Check sheet for the modelled part. Datum: model origin and axes. Units: mm. Face numbers are marked on the shaded views. A direction names the side the tool comes from. Round coordinates to 2 decimals unless told otherwise and drop trailing zeros. Write each loop counter-clockwise with the first axis right and the second up, starting at its lowest first coordinate (ties: lowest second). Pieces come first, ordered by that corner, then holes. Notation, with made-up numbers: M 21.25,87 L 49.25,87 A30 ccw 49.25,114 Z; hole C -40,13.5 d7. An arc over 180 degrees is marked long. One line per item, written item: value.
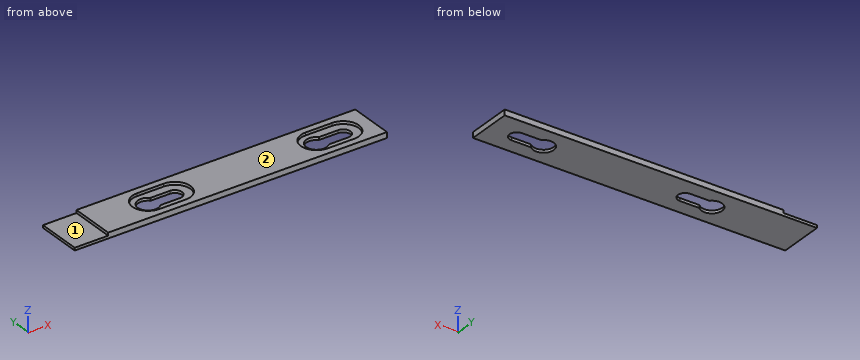
from build123d import *

# Parameters (mm, degrees)
SKETCH_W        = 140
SKETCH_H        = 20
PAD_DEPTH       = 2.5
SKETCH001_W     = 15
SKETCH001_H     = 20
POCKET_DEPTH    = 1.3
POCKET001_DEPTH = 1.25
SKETCH003_R     = 4.6
POCKET002_DEPTH = 1.251


with BuildPart() as part:
    # Sketch → Pad (new body)
    with BuildSketch(Plane.XY):
        with Locations((72, 12)):
            Rectangle(SKETCH_W, SKETCH_H)
    extrude(amount=PAD_DEPTH)

    # Sketch001 → Pocket (cut)
    with BuildSketch(Plane.XY.offset(2.5)):
        with Locations((9.5, 12)):
            Rectangle(SKETCH001_W, SKETCH001_H)
    extrude(amount=-POCKET_DEPTH, mode=Mode.SUBTRACT)

    # Sketch002 → Pocket001 (cut)
    with BuildSketch(Plane.XY.offset(2.5)):
        with BuildLine():
            ThreePointArc((42, 19), (35, 12), (42, 5))
            Line((42, 5), (54, 5))
            ThreePointArc((54, 5), (61, 12), (54, 19))
            Line((42, 19), (54, 19))
        make_face()
        with BuildLine():
            ThreePointArc((117.5, 19), (110.5, 12), (117.5, 5))
            Line((117.5, 5), (129.5, 5))
            ThreePointArc((129.5, 5), (136.5, 12), (129.5, 19))
            Line((117.5, 19), (129.5, 19))
        make_face()
    extrude(amount=-POCKET001_DEPTH, mode=Mode.SUBTRACT)

    # Sketch003 → Pocket002 (cut, through all)
    with BuildSketch(Plane.XY.offset(1.25)):
        with Locations((42, 12)):
            Circle(SKETCH003_R)
        with Locations((117.5, 12)):
            Circle(SKETCH003_R)
        with BuildLine():
            ThreePointArc((54, 8.8), (57.2, 12), (54, 15.2))
            Line((54, 15.2), (44, 15.2))
            ThreePointArc((44, 15.2), (40.8, 12), (44, 8.8))
            Line((54, 8.8), (44, 8.8))
        make_face()
        with BuildLine():
            ThreePointArc((129.5, 8.8), (132.7, 12), (129.5, 15.2))
            Line((129.5, 15.2), (119.5, 15.2))
            ThreePointArc((119.5, 15.2), (116.3, 12), (119.5, 8.8))
            Line((129.5, 8.8), (119.5, 8.8))
        make_face()
    extrude(amount=-POCKET002_DEPTH, mode=Mode.SUBTRACT)


solid = part.part
Q1. Scan lines: line 1 (X direction, y = 12, z = 0.85); line 2 (X direction, y = 13, z = 0.9); line 3 (Y direction, x = 117.5, z = 0.9). Record each from-to range of solid material in increasing order. Write a range as [from, to].
Completed:
line 1: [2, 37.4], [57.2, 112.9], [132.7, 142]
line 2: [2, 37.51], [57.04, 113.01], [132.54, 142]
line 3: [2, 7.4], [16.6, 22]
Q2. Sectioned sample at B-B on y = 12. Enter the section's corners in (x, z).
Completed:
outline: M 2,0 L 37.4,0 L 37.4,1.25 L 35,1.25 L 35,2.5 L 17,2.5 L 17,1.2 L 2,1.2 Z; M 57.2,0 L 112.9,0 L 112.9,1.25 L 110.5,1.25 L 110.5,2.5 L 61,2.5 L 61,1.25 L 57.2,1.25 Z; M 132.7,0 L 142,0 L 142,2.5 L 136.5,2.5 L 136.5,1.25 L 132.7,1.25 Z
Q3. Sectioned sample at A-A on z = 1.9. Enter the section's corners in (x, y).
Completed:
outline: M 17,2 L 142,2 L 142,22 L 17,22 Z; hole M 42,5 L 54,5 A7 ccw 54,19 L 42,19 A7 ccw Z; hole M 117.5,5 L 129.5,5 A7 ccw 129.5,19 L 117.5,19 A7 ccw Z
Q4. Access from +Z, -Z, +X, -X, +Y, -Y to the whole of each face (thin tool, end or side, straight path). Record for the marked faces 1 and 2.
Completed:
face 1: +Z, -X, +Y, -Y
face 2: +Z, +X, -X, +Y, -Y
Q5. Depth check by flat-ended pin: P1, Ø10.5, axis at x = 117.5, y = 12, coming from the +Z side. Enter the tip coordinate at first touch or a pass-through.
Completed:
P1: z = 1.25
